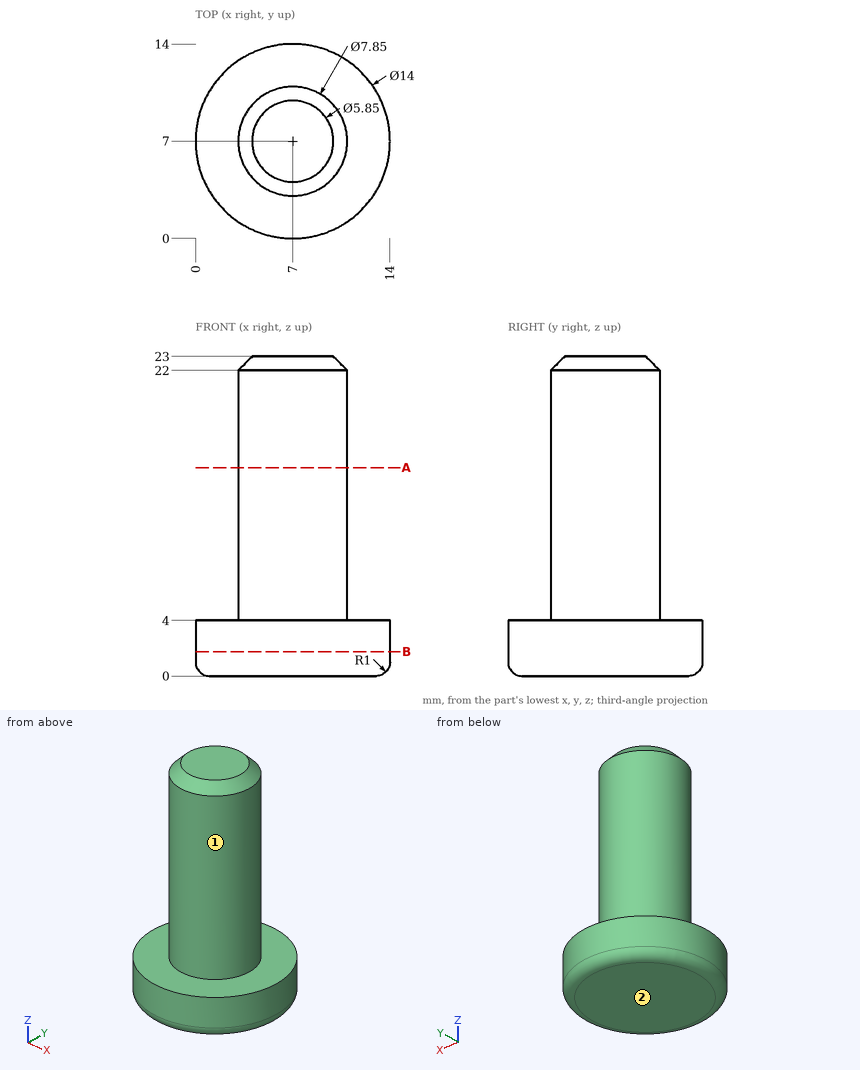
Geometry: see drawing. Coordinates: mm, zero at the bounding-box minimum. A direction names the side the tool comes from. Give positions to 0.01 mm unless a question says otherwise; leave off trailing zeros. Write each loop counter-clockwise with the first axis right and the second up, starting at its lowest first coordinate (ties: lowest second). Pieces come first, ordered by that corner, then holes. Notation, with made-up numbers: M -28,-27 L -12,-27 A26 ccw -12,-10 Z; hole C -31.5,-37 d9. An arc over 180 degrees is marked long. Answer in a Markdown table with one row per item. Add a question column.
(1) Reachability of the marked faces 1 and 2 from +Z, -Z, +X, -X, +Y, -Y: full face, straight path, thin tool, end or side. Return the list, or none.
(2) Section B-B on z = 1.75. Return loops of the section in (x, y), and give its area (3 significant figures).
(3) First-contact query: pin 1 (6 mm diameter, centred on y = 8, z = 9, fed in from +X) (3 decimals); pin 2 (2 mm diameter, centred on x = 1.5, y = 7, fed in from +Z); pin 3 (3 mm diameter, centred on y = 5, z = 18.5, fed in from -X). Flat tips, straight axial feed; report the tip coordinate or a pass-through.
(4) Ray query, line 1 (Z direction, x = 4.5, y = 1.5); line 2 (X direction, y = 12.5, z = 3.25); line 3 (Y direction, x = 4, z = 19.5). Return the intervals inside material, ascending.
(5) Section A-A on z = 15. Return loops of the section in (x, y) (3 decimals), and give its area (3 significant figures).
Result set:
| question | item | result |
|---|---|---|
| 1 | face 1 | +Z |
| 1 | face 2 | -Z, +X, -X, +Y, -Y |
| 2 | outline | C 7,7 d14 |
| 2 | area | 154 mm^2 |
| 3 | pin 1 | stops at x = 10.925 |
| 3 | pin 2 | stops at z = 4 |
| 3 | pin 3 | stops at x = 3.11 |
| 4 | line 1 | z = 0 to 4 |
| 4 | line 2 | x = 2.67 to 11.33 |
| 4 | line 3 | y = 4.47 to 9.53 |
| 5 | outline | C 7,7 d7.85 |
| 5 | area | 48.4 mm^2 |
